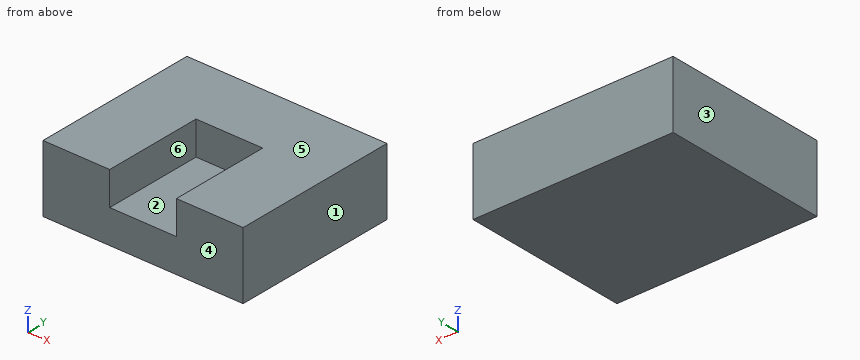
from build123d import *

# Parameters (mm, degrees)
F1_DEPTH = 63.5
F2_W     = 25.4
F2_H     = 12.7
F3_DEPTH = 38.1


with BuildPart() as f1:
    # F0 (on Front) → F1 (new body)
    with BuildSketch(Plane.XZ):
        Polygon((50.8, 12.7), (0, 12.7), (-25.4, 12.7), (-25.4, 0), (-25.4, -12.7), (50.8, -12.7), (50.8, 0), align=None)
    extrude(amount=-F1_DEPTH)

    # F2 (on face) → F3 (cut)
    with BuildSketch(Plane.XZ):
        with Locations((12.7, 6.35)):
            Rectangle(F2_W, F2_H)
    extrude(amount=-F3_DEPTH, mode=Mode.SUBTRACT)


solid = f1.part
Build history of the part. All positions in model axes, mm. Face numbers are marked on the shaded views. A direction names the side the tool comes from. Coordinates: 2 decimals unless noted, no trailing zeros. Order: outer loops, then holes, each group sorted by start corner. A loop starts at its lowest first (then second) coordinate and runs counter-clockwise, first axis right, second up. Notation, with made-up numbers: (62, -5.75) - (92, -5.75) arc R20 ccw to (92, 29.25) - close; hole circle Ø4 at (3.5, 31). An arc over 180 degrees is marked (long way). Write each question's results on one line, items separated by ' | '. Start each with the question number.
Item 1: Mould opens along X. For the marked faces 1, 2, 3 and 4 say: released by +X, released by -X, zero draft, split by the parting line, or undercut.
Item 2: Band-saw the part on A-A on y = 18. Write the cut outline in (x, z), and give its area (3 significant figures).
Item 3: Tool access for the marked faces 5 and 6: list every direction of +Z, -Z, +X, -X, +Y, -Y with a clear straight run to the whole face (end or side of a thin tool).
Item 4: Band-saw the part on C-C on z = 1.25. Write the cut outline in (x, y), and give its area (3 significant figures).
Item 5: Wall check: probe 1 along Y at (x, z) = (1, 7.25); probe 2 along Z at (x, y) = (13, 28); probe 3 along X at (y, z) = (4, 2.25). Give the ranges that are in metal, low to high. Write a range as [from, to].
Item 6: Flat gauge pin, fed straight in: pin 1 (12.5 mm diameter, centred on x = 14.5, y = 21, fed in from +Z). Where does the tip first touch, or does it go through?
Item 7: Band-saw the part on B-B on x = 4. Write the cut outline in (y, z).
Numbers:
1) face 1: released by +X | face 2: undercut | face 3: released by -X | face 4: zero draft
2) outline: (-25.4, -12.7) - (50.8, -12.7) - (50.8, 12.7) - (25.4, 12.7) - (25.4, 0) - (0, 0) - (0, 12.7) - (-25.4, 12.7) - close | area: 1,610 mm^2
3) face 5: +Z, +X, -X, +Y, -Y | face 6: +Z, -Y
4) outline: (-25.4, 0) - (0, 0) - (0, 38.1) - (25.4, 38.1) - (25.4, 0) - (50.8, 0) - (50.8, 63.5) - (-25.4, 63.5) - close | area: 3,870 mm^2
5) probe 1: [38.1, 63.5] | probe 2: [-12.7, 0] | probe 3: [-25.4, 0], [25.4, 50.8]
6) pin 1: z = 0
7) outline: (0, -12.7) - (63.5, -12.7) - (63.5, 12.7) - (38.1, 12.7) - (38.1, 0) - (0, 0) - close
